from build123d import *

# Parameters (mm, degrees)
M4X0_7_TAPPED_HOLE1_D     = 3.3
M4X0_7_TAPPED_HOLE1_DEPTH = 12


with BuildPart() as part:
    # Sketch1 → Revolve1 (revolve)
    with BuildSketch(Plane.XY, mode=Mode.PRIVATE) as revolve1_sk:
        Polygon((-2, 1.740967464), (2, 1.740967464), (3, 5.740967464), (6, 5.740967464), (6, -9.259032536), (-6, -9.259032536), (-6, 5.740967464), (-3, 5.740967464), align=None)
    revolve(revolve1_sk.sketch.rotate(Axis((-24.289514567, -14.259032536, 0), (1, 0, 0)), 90), axis=Axis((-24.289514567, -14.259032536, 0), (1, 0, 0)))

    # M4x0.7 Tapped Hole1
    with Locations(Plane(origin=(0.112968309, 0.556468612, 6.041599599), x_dir=(0, -0.377599974944, 0.925968821787), z_dir=(0, 0.925968821787, 0.377599974944))):
        with Locations((0, 0)):
            Hole(M4X0_7_TAPPED_HOLE1_D / 2, depth=M4X0_7_TAPPED_HOLE1_DEPTH)


solid = part.part
The listing builds one solid part. Answer for the finished solid, in the listing's coordinates (mm). A direction names the side the tool comes from. Round coordinates to 2 decimals unless told otherwise and drop trailing zeros. Write each loop counter-clockwise with the first axis right and the second up, starting at its lowest first coordinate (ties: lowest second). Pieces come first, ordered by that corner, then holes. Notation, with made-up numbers: (15, 57) - (29, 57) arc R19 ccw to (29, 76) - close; hole circle Ø3 at (-34.5, 30). An arc over 180 degrees is marked (long way). Use one line per item in the form item = value. Start each with the question number.
Item 1: A tool of negligible diameter and unlimited length cuts with its end or side. For faces 1 (the cylindrical face through (-0.084, -19.216, -0.651)), 2 (the cylindrical face through (0.028, -30.123, -2.083)), from which of +Z, -Z, +X, -X, +Y, -Y can it reach the whole face along a straight path? Write none if from no direction.
Item 2: A cutting plane is placed at A-A (x = 2.5). Write down the section's boundary in (y, z), plus the area to 3 significant figures.
Item 3: A cutting plane is placed at B-B (x = -0.5). Write down the section's boundary in (y, z), plus the area to 3 significant figures.
Item 4: Flat-ended cylindrical pins translate along their axes: pin 1 Ø1 at (x, z) = (4.5, 14) entering from -Y; pin 2 Ø3 at (x, y) = (3.5, -6.5) entering from -Z. Find the tip coordinate at first contact, or state that the pin passes through.
Item 5: Find the intervals of material crossed by line 1 (Y direction, x = 0.75, z = 0); line 2 (Y direction, x = -3.25, z = 0); line 3 (X direction, y = 3.5, z = 2.5), in increasing order. Write a range as [from, to].
Item 6: A cutting plane is placed at C-C (x = -4.75). Write down the section's boundary in (y, z), plus the area to 3 significant figures.
Item 7: Determine the mould class of faces 3 (the conical face through (2.063, -19.14, 15.5)), 4 (the cylindrical face through (-4.479, 5.265, -4.336)), 5 (the flat face through (6, -10, 4)) for opening direction X: +X half, -X half, draft (parallel to the pull), parting line (faces both ways), or undercut.
The answers:
q1.face_1 = +X, -X
q1.face_2 = none
q2.outline = circle Ø36 at (-14.26, 0); hole circle Ø10 at (-14.26, 0)
q2.area = 939 mm^2
q3.outline = (-10.43, 3.22) - (-0.09, 7.43) arc R16 ccw (long way) to (1.07, 4.6) - (-9.27, 0.38) arc R5 cw (long way) to start
q3.area = 692 mm^2
q4.pin_1 = -29.02
q4.pin_2 = -19
q5.line_1 = [-30.26, -19.26], [-9.26, 1.74]
q5.line_2 = [-34.26, -19.26], [-9.26, 5.74]
q5.line_3 = [-6, -2.48], [2.48, 6]
q6.outline = circle Ø40 at (-14.26, 0); hole circle Ø10 at (-14.26, 0)
q6.area = 1,180 mm^2
q7.face_3 = undercut
q7.face_4 = draft
q7.face_5 = +X half
